Autodesk Inventor part; units mm, degrees
ref_plane "YZ Plane" through (0, 0, 0) normal (1, 0, 0) x (0, 1, 0)
ref_plane "XZ Plane" through (0, 0, 0) normal (0, 1, 0) x (-1, 0, 0)
ref_plane "XY Plane" through (0, 0, 0) normal (0, 0, 1) x (1, 0, 0)
sketch "Sketch1" plane through (0, 0, 0) normal (0, 0, 1) x (1, 0, 0)
  line L0 (-15.75, 17) -> (15.75, 17)
  line L1 (15.75, 17) -> (15.75, -17)
  line L2 (15.75, -17) -> (-15.75, -17)
  line L3 (-15.75, -17) -> (-15.75, 17)
  point P0 (0, 0)
  point P1 (15.75, 0)
  point P2 (0, 17)
  dimension "d0" = 34
  dimension "d1" = 31.5
extrude "Extrusion1" add sketch "Sketch1" along normal blind 2
sketch "Sketch2" plane through (0, 0, 2) normal (0, 0, 1) x (1, 0, 0)
  line L0 (-11.5, 8) -> (-15.75, 8)
  line L1 (-15.75, 8) -> (-15.75, -13)
  line L2 (-15.75, -13) -> (-11.5, -13)
  line L3 (-11.5, -13) -> (-11.5, 8)
  line L4 (11.5, 8) -> (15.75, 8)
  line L5 (15.75, 8) -> (15.75, -13)
  line L6 (15.75, -13) -> (11.5, -13)
  line L7 (11.5, -13) -> (11.5, 8)
  line L8 (15.75, -13) -> (-15.75, -13)
  line L9 (-15.75, -13) -> (-15.75, -17)
  line L10 (-15.75, -17) -> (15.75, -17)
  line L11 (15.75, -17) -> (15.75, -13)
  line L12 (-15.75, 17) -> (-15.75, -17)
  line L13 (15.75, 17) -> (-15.75, 17)
  line L14 (15.75, -17) -> (15.75, 17)
  line L15 (-15.75, -17) -> (15.75, -17)
  point P0 (0, 0)
  dimension "d4" = 23
  dimension "d5" = 4
  dimension "d67" = 21
extrude "Extrusion2" add sketch "Sketch2" along normal blind 12 contours L3 L2 L1 L0 | L8 L6 L11 L10 L9 L2 | L7 L4 L5 L6
sketch "Sketch8" plane through (-11.5, -13, 2) normal (0, 1, 0) x (1, 0, 0)
  circle A0 centre (6, -6) radius 6 construction
  circle A1 centre (17, -6) radius 6 construction
  line L0 (0, 0) -> (0, -12) construction
  line L1 (23, -12) -> (0, -12) construction
  line L2 (0, 0) -> (23, 0) construction
  line L3 (23, 0) -> (23, -12) construction
  circle A2 centre (6, -6) radius 1.675
  circle A3 centre (17, -6) radius 1.675
  point P0 (11.5, 2)
  dimension "d29" = 3.35
extrude "Extrusion8" cut sketch "Sketch8" against normal through all
sketch "Sketch9" plane through (-11.5, -13, 2) normal (0, 1, 0) x (1, 0, 0)
  line L0 (3.075, -8.925) -> (8.925, -8.925)
  line L1 (8.925, -8.925) -> (8.925, -3.075)
  line L2 (8.925, -3.075) -> (3.075, -3.075)
  line L3 (3.075, -3.075) -> (3.075, -8.925)
  line L4 (14.075, -8.925) -> (19.925, -8.925)
  line L5 (19.925, -8.925) -> (19.925, -3.075)
  line L6 (19.925, -3.075) -> (14.075, -3.075)
  line L7 (14.075, -3.075) -> (14.075, -8.925)
  circle A0 centre (6, -6) radius 1.675
  circle A1 centre (17, -6) radius 1.675
  point P0 (11.5, 2)
  point P1 (6, -3.075)
  point P2 (17, -3.075)
  point P3 (3.075, -6)
  point P4 (14.075, -6)
  dimension "d32" = 5.85
extrude "Extrusion9" cut sketch "Sketch9" against normal blind 2.15
sketch "Sketch10" plane through (0, 0, 0) normal (0, 0, -1) x (-1, 0, 0)
  line L0 (-15.75, 17) -> (15.75, 17)
  line L1 (15.75, 17) -> (15.75, -12)
  line L2 (15.75, -12) -> (-15.75, -12)
  line L3 (-15.75, -12) -> (-15.75, 17)
  line L4 (-15.75, -17) -> (15.75, -17)
  line L5 (15.75, 17) -> (-15.75, 17)
  line L6 (-15.75, 17) -> (-15.75, -17)
  point P0 (0, 0)
  point P1 (0, 17)
  point P2 (15.75, 2.5)
  dimension "d36" = 29
extrude "Extrusion10" add sketch "Sketch10" along normal blind 3
sketch "Sketch16" plane through (15.75, -17, 14) normal (1, 0, 0) x (0, 0, -1)
  line L0 (1.75, 8) -> (10.25, 8)
  line L1 (10.25, 8) -> (10.25, 4)
  line L2 (10.25, 4) -> (1.75, 4)
  line L3 (1.75, 4) -> (1.75, 8)
  line L4 (12, 4) -> (0, 4)
  point P0 (14, 17)
  point P1 (6, 8)
  point P2 (6, 4)
  point P3 (6, 4)
  dimension "d62" = 8.5
  dimension "d63" = 4
extrude "Extrusion16" cut sketch "Sketch16" against normal through all
sketch "Sketch20" plane through (-15.75, 8, 2) normal (0, 1, 0) x (1, 0, 0)
  circle A0 centre (1.5, -6) radius 1.25
  circle A1 centre (30, -6) radius 1.25
  line L0 (4.25, -12) -> (0, -12)
  line L1 (4.25, 0) -> (4.25, -12)
  line L2 (27.25, 0) -> (27.25, -12)
  point P0 (15.75, 2)
  point P1 (4.25, -6)
  dimension "d90" = 2.5
  dimension "d92" = 1.5
  dimension "d93" = 1.5
extrude "Extrusion20" cut sketch "Sketch20" against normal blind 10
sketch "Sketch21" plane through (-15.75, -17, 14) normal (-1, 0, 0) x (0, 0, 1)
  line L0 (-17, 12.5) -> (-10.25, 12.5)
  line L1 (-10.25, 12.5) -> (-10.25, 8.5)
  line L2 (-10.25, 8.5) -> (-17, 8.5)
  line L3 (-17, 8.5) -> (-17, 12.5)
  line L4 (-14, 0) -> (0, 0)
  line L5 (-17, 5) -> (-17, 34)
  point P0 (-14, 17)
  point P1 (-17, 7)
  point P2 (-10.25, 8)
  dimension "d96" = 8.5
  dimension "d100" = 4
extrude "Extrusion21" add sketch "Sketch21" along normal blind 5.35
sketch "Sketch24" plane through (15.75, -17, 14) normal (1, 0, 0) x (0, 0, -1)
  line L0 (10.25, 12.5) -> (17, 12.5)
  line L1 (17, 12.5) -> (17, 8.5)
  line L2 (17, 8.5) -> (10.25, 8.5)
  line L3 (10.25, 8.5) -> (10.25, 12.5)
  line L4 (17, 34) -> (17, 5)
  line L5 (14, 0) -> (0, 0)
  point P0 (14, 17)
  point P1 (17, 7)
  point P2 (10.25, 8)
  dimension "d107" = 8.5
  dimension "d108" = 4
extrude "Extrusion24" add sketch "Sketch24" along normal blind 5.35
sketch "Sketch22" plane through (-15.75, -4.5, 3.75) normal (0, 1, 0) x (1, 0, 0)
  circle A0 centre (-2.675, 3.375) radius 1.175
  line L0 (-5.35, 0) -> (-5.35, 6.75)
  line L1 (0, 0) -> (-5.35, 0)
  circle A1 centre (34.175, 3.375) radius 1.175
  line L2 (31.5, 0) -> (36.85, 0)
  point P0 (15.75, 3.75)
  point P1 (-5.35, 3.375)
  point P2 (-2.675, 0)
  point P3 (34.175, 0)
  dimension "d101" = 2.35
extrude "Extrusion22" cut sketch "Sketch22" against normal through all
sketch "Sketch23" plane through (-15.75, -4.5, 3.75) normal (0, 1, 0) x (1, 0, 0)
  circle A0 centre (-2.675, 3.375) radius 2.175
  circle A1 centre (-2.675, 3.375) radius 1.175
  circle A2 centre (34.175, 3.375) radius 2.175
  circle A3 centre (34.175, 3.375) radius 1.175
  point P0 (15.75, 3.75)
  dimension "d104" = 4.35
extrude "Extrusion23" cut sketch "Sketch23" against normal blind 2
sketch "Sketch25" plane through (15.75, -17, 14) normal (1, 0, 0) x (0, 0, -1)
  line L0 (3.825, 22.075) -> (8.175, 22.075)
  line L1 (8.175, 22.075) -> (8.175, 20)
  line L2 (8.175, 20) -> (3.825, 20)
  line L3 (3.825, 20) -> (3.825, 22.075)
  line L4 (12, 25) -> (0, 25)
  point P0 (14, 17)
  point P1 (6, 25)
  point P2 (6, 22.075)
  dimension "d111" = 5
  dimension "d112" = 2.075
  dimension "d113" = 4.35
extrude "Extrusion25" cut sketch "Sketch25" against normal through all
sketch "Sketch26" plane through (0, 0, 2) normal (0, 0, 1) x (1, 0, 0)
  line L0 (-15.75, 17) -> (15.75, 17)
  line L1 (15.75, 17) -> (15.75, 8)
  line L2 (15.75, 8) -> (-15.75, 8)
  line L3 (-15.75, 8) -> (-15.75, 17)
  line L4 (11.5, 8) -> (15.75, 8)
  line L5 (15.75, 8) -> (15.75, 17)
  line L6 (-15.75, 17) -> (-15.75, 8)
  line L7 (15.75, 17) -> (-15.75, 17)
  point P0 (0, 0)
extrude "Extrusion26" cut sketch "Sketch26" against normal through all
sketch "Sketch27" plane through (0, 0, 0) normal (0, 0, -1) x (-1, 0, 0)
  line L0 (-15.75, -17) -> (15.75, -17)
  line L1 (15.75, -12) -> (-15.75, -12)
  line L2 (15.75, -17) -> (-15.75, -17)
  line L3 (-15.75, -17) -> (-15.75, -12)
  line L4 (-15.75, -12) -> (15.75, -12)
  line L5 (15.75, -12) -> (15.75, -17)
  point P0 (0, 0)
extrude "Extrusion27" cut sketch "Sketch27" against normal blind 0.3
equation "\"d1\" = servo_D"
equation "\"d4\" = servo_A"
equation "\"d5\" = bot_mat"
equation "\"d67\" = servo_E"
equation "\"d6\" = servo_B"
equation "\"d33\" = nut_B"
equation "\"d92\" = servo_L"
equation "\"d93\" = d92"
equation "\"d109\" = d97"
equation "\"d112\" = nut_B_1 + Tolerance"
equation "\"d113\" = nut_A_1"
equation "\"bot_mat\" = 4"
properties part number "HIP"
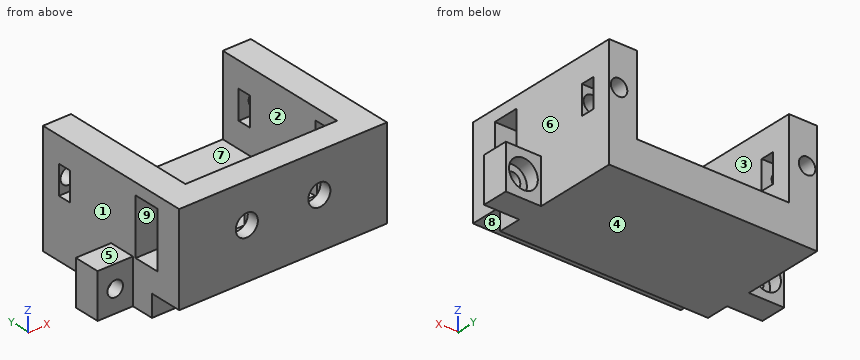
Geometry check sheet. Reference: the model listing, model coordinates, mm. Face numbers are marked on the shaded views. A direction names the side the tool comes from. Give positions to 0.01 mm unless a question says otherwise; leave off trailing zeros. Loops run counter-clockwise (first coordinate to the right, second up) from the corner with the lowest first, then second, coordinate; pieces in that order, holes last.
(1) Section check D-D on z = 8. Count the separate pieces of the cut face and the enclosed holes in it, then the cut area to 3 significant figures.
From the geometry:
separate pieces: 9
enclosed holes: 0
area: 176 mm2
(2) Thickness scan on L1, parallel to Y at x = 14, z = 6.5 (3 decimals); L2, parallel to X at y = -16.25, z = 8 (3 decimals); L3, parallel to Z at x = 14, y = -12.5. Record the ranges inside material, lowest first.
From the geometry:
L1: y = -17 to -13, -9 to 3, 5.075 to 8
L2: x = -15.75 to -7.175, -3.825 to 3.825, 7.175 to 15.75
L3: z = 0.3 to 3.75, 12.25 to 14
(3) Section check B-B on y = -0.75. Record the cut outline in (x, z), then the cut area to 3 significant figures.
From the geometry:
outline: (-15.75, -3) - (15.75, -3) - (15.75, 14) - (11.5, 14) - (11.5, 2) - (-11.5, 2) - (-11.5, 14) - (-15.75, 14) - close; hole circle Ø2.5 at (-14.25, 8); hole circle Ø2.5 at (14.25, 8)
area: 250 mm2
(4) Section check A-A on x = 5.5. Record the cut outline in (y, z) (3 decimals), then the cut area to 3 significant figures.
From the geometry:
outline: (-17, 0.3) - (-12, 0.3) - (-12, -3) - (8, -3) - (8, 2) - (-13, 2) - (-13, 5.075) - (-15.15, 5.075) - (-15.15, 6.325) - (-17, 6.325) - close; (-17, 9.675) - (-15.15, 9.675) - (-15.15, 10.925) - (-13, 10.925) - (-13, 14) - (-17, 14) - close
area: 138 mm2
(5) Depth check by flat-ended pin: pin 1 Ø2 at (x, z) = (18.425, 0.375) entering from +Y; pin 2 Ø1.7 at (y, z) = (-14.5, 8.5) entering from -X; pin 3 Ø1.6 at (x, z) = (-18, -1) entering from -Y; pin 4 Ø6 at (x, z) = (2, 11) entering from +Y. Enter the tip coordinate at first touch or a pass-through.
From the geometry:
pin 1: passes through
pin 2: stops at x = -15.75
pin 3: stops at y = -8.5
pin 4: stops at y = -13
(6) Release check for a two-part mould opening along X. For the marked faces 1, 2, 3 and 4 record: released by +X, released by -X, zero draft, split by the parting line, or undercut.
From the geometry:
face 1: released by -X
face 2: undercut
face 3: undercut
face 4: zero draft
(7) Section check C-C on x = -14.25. Record the cut outline in (y, z) (3 decimals).
From the geometry:
outline: (-17, 0.3) - (-12, 0.3) - (-12, -3) - (8, -3) - (8, 6.75) - (5.075, 6.75) - (5.075, 5.825) - (3, 5.825) - (3, 6.75) - (-2, 6.75) - (-2, 9.25) - (3, 9.25) - (3, 10.175) - (5.075, 10.175) - (5.075, 9.25) - (8, 9.25) - (8, 14) - (-17, 14) - close; hole (-13, 3.75) - (-9, 3.75) - (-9, 12.25) - (-13, 12.25) - close
(8) Set-up check for the marked faces 5, 6, 7, 8 and 9: record each of +Z, -Z, +X, -X, +Y, -Y from which the full face is reachable in a straight line by a thin tool's end or side.
From the geometry:
face 5: +Z, -X, +Y, -Y
face 6: +Z, +X
face 7: +Z, +Y
face 8: -Z, +X, -X, -Y
face 9: +X, -X
